Could you check a few things on this model? Use its own coordinates, in mm. Face numbers are marked on the shaded views. A direction names the side the tool comes from. Coordinates: 2 decimals unless noted, no trailing zeros. Loops run counter-clockwise (first coordinate to the right, second up) from the corner with the lowest first, then second, coordinate; pieces in that order, holes last. Notation, with made-up numbers: (82.5, -30.5) -> (106.5, -30.5) arc R24 cw to (106.5, -0.5) -> close; hole circle Ø8 at (-27, 17.5). An arc over 180 degrees is marked (long way). One line per question, with ' | ' between items.
from build123d import *

# Parameters (mm, degrees)
SKETCH1_R           = 9
SKETCH1_R_2         = 3
BOSS_EXTRUDE2_DEPTH = 10


with BuildPart() as part:
    # Sketch1 → Boss-Extrude2 (new body)
    with BuildSketch(Plane.XY):
        with BuildLine():
            Line((-49.041889066, 5.908846518), (-14.079486813, 12.073661346))
            ThreePointArc((-14.079486813, 12.073661346), (-8.205154011, 14.211743632), (-3.416354035, 18.230023925))
            Line((-3.416354035, 18.230023925), (19.403733341, 45.42594504))
            ThreePointArc((19.403733341, 45.42594504), (27, 46.765371804), (29.638155725, 39.517098522))
            Line((29.638155725, 39.517098522), (17.495840849, 6.15636258))
            ThreePointArc((17.495840849, 6.15636258), (16.410308023, 0), (17.495840849, -6.15636258))
            Line((17.495840849, -6.15636258), (29.638155725, -39.517098522))
            ThreePointArc((29.638155725, -39.517098522), (27, -46.765371804), (19.403733341, -45.42594504))
            Line((19.403733341, -45.42594504), (-3.416354035, -18.230023925))
            ThreePointArc((-3.416354035, -18.230023925), (-8.205154011, -14.211743632), (-14.079486813, -12.073661346))
            Line((-14.079486813, -12.073661346), (-49.041889066, -5.908846518))
            ThreePointArc((-49.041889066, -5.908846518), (-54, 0), (-49.041889066, 5.908846518))
        make_face()
        Circle(SKETCH1_R, mode=Mode.SUBTRACT)
        with Locations((-48, 0)):
            Circle(SKETCH1_R_2, mode=Mode.SUBTRACT)
        with Locations((24, 41.569219382)):
            Circle(SKETCH1_R_2, mode=Mode.SUBTRACT)
        with Locations((24, -41.569219382)):
            Circle(SKETCH1_R_2, mode=Mode.SUBTRACT)
        with BuildLine():
            Line((-40.269689417, 4.409342161), (-13.089403061, 9.201959989))
            ThreePointArc((-13.089403061, 9.201959989), (-10.726679899, 8.24313144), (-10.560539529, 5.698684484))
            ThreePointArc((-10.560539529, 5.698684484), (-12, 0), (-10.560539529, -5.698684484))
            ThreePointArc((-10.560539529, -5.698684484), (-10.726679899, -8.24313144), (-13.089403061, -9.201959989))
            Line((-13.089403061, -9.201959989), (-40.269689417, -4.409342161))
            ThreePointArc((-40.269689417, -4.409342161), (-41.866838007, -3.351249763), (-42.180666993, -1.461288252))
            ThreePointArc((-42.180666993, -1.461288252), (-42, 0), (-42.180666993, 1.461288252))
            ThreePointArc((-42.180666993, 1.461288252), (-41.866838007, 3.351249763), (-40.269689417, 4.409342161))
        make_face(mode=Mode.SUBTRACT)
        with BuildLine():
            Line((23.953447034, 32.669902957), (14.513832645, 6.734775577))
            ThreePointArc((14.513832645, 6.734775577), (12.502101183, 5.168011571), (10.215475296, 6.296353268))
            ThreePointArc((10.215475296, 6.296353268), (6, 10.392304845), (0.345064233, 11.995037752))
            ThreePointArc((0.345064233, 11.995037752), (-1.775421284, 13.41114301), (-1.424429584, 15.936735566))
            Line((-1.424429584, 15.936735566), (16.316242383, 37.079245118))
            ThreePointArc((16.316242383, 37.079245118), (18.031151575, 37.933370172), (19.824820748, 37.260173291))
            ThreePointArc((19.824820748, 37.260173291), (21, 36.373066959), (22.355846246, 35.798885039))
            ThreePointArc((22.355846246, 35.798885039), (23.835686433, 34.582120409), (23.953447034, 32.669902957))
        make_face(mode=Mode.SUBTRACT)
        with BuildLine():
            Line((16.316242383, -37.079245118), (-1.424429584, -15.936735566))
            ThreePointArc((-1.424429584, -15.936735566), (-1.775421284, -13.41114301), (0.345064233, -11.995037752))
            ThreePointArc((0.345064233, -11.995037752), (6, -10.392304845), (10.215475296, -6.296353268))
            ThreePointArc((10.215475296, -6.296353268), (12.502101183, -5.168011571), (14.513832645, -6.734775577))
            Line((14.513832645, -6.734775577), (23.953447034, -32.669902957))
            ThreePointArc((23.953447034, -32.669902957), (23.835686433, -34.582120409), (22.355846246, -35.798885039))
            ThreePointArc((22.355846246, -35.798885039), (21, -36.373066959), (19.824820748, -37.260173291))
            ThreePointArc((19.824820748, -37.260173291), (18.031151575, -37.933370172), (16.316242383, -37.079245118))
        make_face(mode=Mode.SUBTRACT)
    extrude(amount=BOSS_EXTRUDE2_DEPTH)


solid = part.part
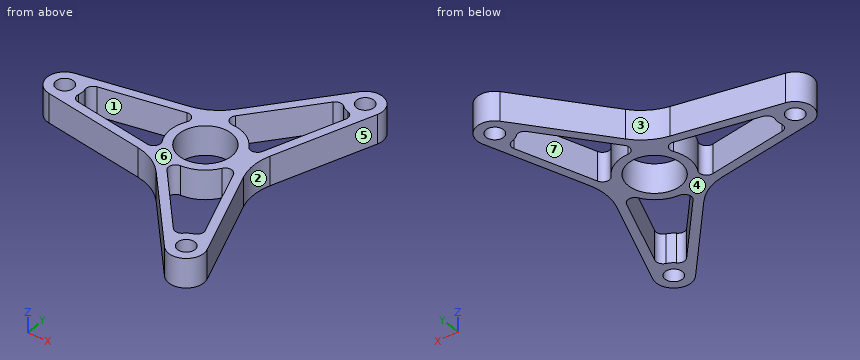
1) If we section it at C-C on z = 7.5: Give the number of separate pieces and of enclosed holes in the cut face, and give its area (3 significant figures).
Data:
separate pieces: 1 | enclosed holes: 7 | area: 1,230 mm²
2) On a 3-axis mill with a long thin cutter (end or side, diameter ignored), from which of +Z, -Z, +X, -X, +Y, -Y can I reach the whole of each face in a straight line? I mean the marked faces 5, 6 and 7. Say none if no direction works.
Data:
face 5: +Z, -Z, +X | face 6: +Z, +X, -X, +Y, -Y | face 7: +Z, -Z
3) If we section it at A-A on y = 0: Please give me the cut outline in (x, z).
Data:
outline: (-54, 0) -> (-51, 0) -> (-51, 10) -> (-54, 10) -> close; (-45, 0) -> (-42, 0) -> (-42, 10) -> (-45, 10) -> close; (-12, 0) -> (-9, 0) -> (-9, 10) -> (-12, 10) -> close; (9, 0) -> (16.41, 0) -> (16.41, 10) -> (9, 10) -> close
4) We'd pull the mould along X, two halves only. Please class the marked faces 1, 2, 3 and 4: pulls with the +X half, pulls with the -X half, needs draft (parallel to the pull), parting line crosses it, or undercut.
Data:
face 1: undercut | face 2: pulls with the +X half | face 3: pulls with the -X half | face 4: needs draft
5) If we section it at B-B on x = -47: Please give me the cut outline in (y, z).
Data:
outline: (-6.27, 0) -> (-2.83, 0) -> (-2.83, 10) -> (-6.27, 10) -> close; (2.83, 0) -> (6.27, 0) -> (6.27, 10) -> (2.83, 10) -> close
6) If we section it at D-D on x = -26.5: Please give me the cut outline in (y, z).
Data:
outline: (-9.88, 0) -> (-6.84, 0) -> (-6.84, 10) -> (-9.88, 10) -> close; (6.84, 0) -> (9.88, 0) -> (9.88, 10) -> (6.84, 10) -> close
7) I need wall thicknesses on line 1 along Y through (x, z) = (0, 7.5); line 2 along Y through (x, z) = (5, 4); line 3 along X through (y, z) = (30, 5.5). Which ranges of each line are inside material? Lowest first, please. Write a range as from..to.
Data:
line 1: -22.3..-17.63, -12.03..-9, 9..12.03, 17.63..22.3 | line 2: -28.26..-23.59, -10.91..-7.48, 7.48..10.91, 23.59..28.26 | line 3: 6.46..10.38, 22.98..26.17
8) I'm going to push flat-ended pins straight in: pin 1 Ø1.5 at (x, z) = (-18.5, 3.5) entering from +Y; pin 2 Ø20.5 at (x, y) = (0, 0) entering from +Z; pin 3 Ø5 at (x, z) = (-21, 8.5) entering from -Y; pin 4 Ø4 at (y, z) = (19, 2) entering from -X. Where does each tip first touch, or does it pass through?
Data:
pin 1: y = 11.43 | pin 2: z = 10 | pin 3: y = -11.29 | pin 4: x = -4.55
